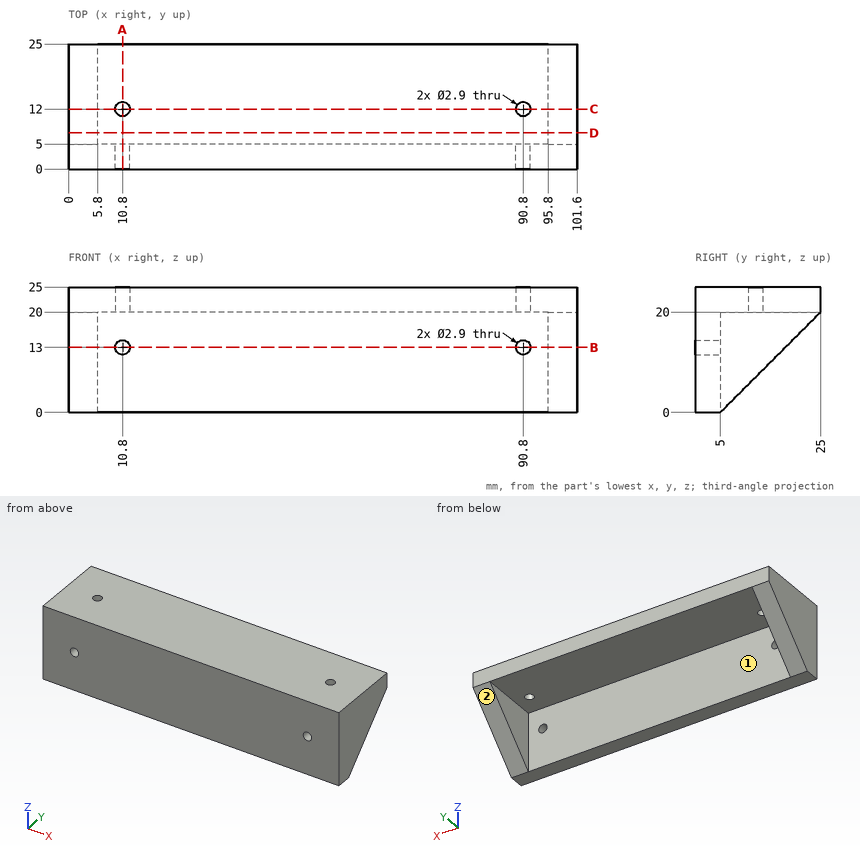
Input: dimensioned drawing with shaded views. Units: mm. Origin: part minimum x, y, z. A direction names the side the tool comes from. Coordinates: 2 decimals unless noted, no trailing zeros. Loops run counter-clockwise (first coordinate to the right, second up) from the corner with the lowest first, then second, coordinate; pieces in that order, holes last. Notation, with made-up numbers: (72.5, 73.25) -> (121.5, 73.25) arc R21 ccw to (121.5, 94.25) -> close; hole circle Ø1 at (-23, -4.75). An arc over 180 degrees is marked (long way). Use a Markdown table: item, result. Add a question column.
(1) Section query D-D, the plane y = 7.25. Return loops of the section in (x, z), plus the area to 3 significant figures.
(2) Pin query (flat end, axial travel): pin 1 Ø5 at (x, z) = (36, 2.5) entering from -Y; pin 2 Ø10 at (x, y) = (51, 14.5) entering from -Z; pin 3 Ø2.5 at (x, z) = (90.8, 13) entering from +Y (3 decimals). Return the tip coordinate at first contact, or that it passes through.
(3) Section query B-B, the plane z = 13. Return loops of the section in (x, y), plus the area to 3 significant figures.
(4) Line query: line 1 along X through (y, z) = (2.9, 13); line 2 along X through (y, z) = (8, 15); line 3 along Y through (x, z) = (90.8, 22.2). Output: solid intervals per line, ascending.
(5) Section query C-C, the plane y = 12. Return loops of the section in (x, z).
(6) Access query for the marked faces 1 and 2. Directions: +Z, -Z, +X, -X, +Y, -Y. A direction counts if a zero-diameter tool reaches every point of the face in a straight line with its end or side. Return the directions, or none.
(7) Section query A-A, the plane x = 10.8. Return loops of the section in (y, z), plus the area to 3 significant figures.
Answer:
| question | item | result |
|---|---|---|
| 1 | outline | (0, 2.25) -> (5.8, 2.25) -> (5.8, 20) -> (95.8, 20) -> (95.8, 2.25) -> (101.6, 2.25) -> (101.6, 25) -> (0, 25) -> close |
| 1 | area | 714 mm^2 |
| 2 | pin 1 | stops at y = 0 |
| 2 | pin 2 | stops at z = 20 |
| 2 | pin 3 | passes through |
| 3 | outline | (0, 0) -> (9.35, 0) -> (9.35, 5) -> (5.8, 5) -> (5.8, 18) -> (0, 18) -> close; (12.25, 0) -> (89.35, 0) -> (89.35, 5) -> (12.25, 5) -> close; (92.25, 0) -> (101.6, 0) -> (101.6, 18) -> (95.8, 18) -> (95.8, 5) -> (92.25, 5) -> close |
| 3 | area | 630 mm^2 |
| 4 | line 1 | x = 0 to 9.35, 12.25 to 89.35, 92.25 to 101.6 |
| 4 | line 2 | x = 0 to 5.8, 95.8 to 101.6 |
| 4 | line 3 | y = 0 to 10.55, 13.45 to 25 |
| 5 | outline | (0, 7) -> (5.8, 7) -> (5.8, 20) -> (9.35, 20) -> (9.35, 25) -> (0, 25) -> close; (12.25, 20) -> (89.35, 20) -> (89.35, 25) -> (12.25, 25) -> close; (92.25, 20) -> (95.8, 20) -> (95.8, 7) -> (101.6, 7) -> (101.6, 25) -> (92.25, 25) -> close |
| 6 | face 1 | -Z, +Y |
| 6 | face 2 | -Z, +X, -X, +Y |
| 7 | outline | (0, 0) -> (5, 0) -> (5, 11.55) -> (0, 11.55) -> close; (0, 14.45) -> (5, 14.45) -> (5, 20) -> (10.55, 20) -> (10.55, 25) -> (0, 25) -> close; (13.45, 20) -> (25, 20) -> (25, 25) -> (13.45, 25) -> close |
| 7 | area | 196 mm^2 |
